from build123d import *

# Parameters (mm, degrees)
SKETCH_1_W             = 56
SKETCH_1_H             = 88
EXTRUDE_1_DEPTH        = 2.7
FILLET_1_R             = 1
SKETCH_8_R             = 1.6
SKETCH_8_R_2           = 1.75
CUT_EXTRUDE_1_DEPTH    = 10
CHAMFER_1_SIZE         = 6
SKETCH_16_R            = 3
EXTRUDE_3_DEPTH        = 1
HOLE_WIZARD_M4_1_D     = 3.3
HOLE_WIZARD_M4_1_DEPTH = 10.1
HOLE_WIZARD_M4_1_TIP   = 0.991420021
SKETCH_11_W            = 6
SKETCH_11_H            = 6
EXTRUDE_2_DEPTH        = 3.3
HOLE_WIZARD_M3_1_D     = 2.5
HOLE_WIZARD_M3_1_DEPTH = 7.5
HOLE_WIZARD_M3_1_TIP   = 0.751075774
SKETCH_14_W            = 30
SKETCH_14_H            = 47
CUT_EXTRUDE_2_DEPTH    = 10
FILLET_2_R             = 2
SKETCH_15_W            = 20
SKETCH_15_H            = 2.7
CUT_EXTRUDE_3_DEPTH    = 5
CHAMFER_2_SIZE         = 0.5
FILLET_3_R             = 2


with BuildPart() as part:
    # 草图1 → 凸台-拉伸1 (new body)
    with BuildSketch(Plane.XY):
        Rectangle(SKETCH_1_W, SKETCH_1_H)
    extrude(amount=EXTRUDE_1_DEPTH)

    # 圆角1
    fillet_1_edges = [part.edges().sort_by_distance(p)[0] for p in [
        (28, -44, 1.35),
        (28, 44, 1.35),
    ]]
    fillet(fillet_1_edges, radius=FILLET_1_R)

    # 草图8 → 切除-拉伸1 (cut)
    with BuildSketch(Plane(origin=(0, 0, 0), x_dir=(-1, 0, 0), z_dir=(0, 0, -1))):
        with Locations((-24, 41)):
            Circle(SKETCH_8_R)
        with Locations((20, 41)):
            Circle(SKETCH_8_R_2)
        with Locations((-24, -41)):
            Circle(SKETCH_8_R)
        with Locations((20, -41)):
            Circle(SKETCH_8_R_2)
    extrude(amount=-CUT_EXTRUDE_1_DEPTH, mode=Mode.SUBTRACT)

    # 倒角1
    chamfer_1_edges = [part.edges().sort_by_distance(p)[0] for p in [
        (-28, -44, 1.35),
        (-28, 44, 1.35),
    ]]
    chamfer(chamfer_1_edges, length=CHAMFER_1_SIZE)

    # 草图16 → 凸台-拉伸3 (add)
    with BuildSketch(Plane(origin=(0, 0, 0), x_dir=(-1, 0, 0), z_dir=(0, 0, -1))):
        with Locations((22.2, -20.7)):
            Circle(SKETCH_16_R)
        with Locations((-20.2, 30.7)):
            Circle(SKETCH_16_R)
    extrude(amount=EXTRUDE_3_DEPTH)

    # M4 螺纹孔1
    with Locations(Plane.XY.offset(2.7)):
        with Locations((20.2, 30.7), (-22.2, -20.7)):
            Hole(HOLE_WIZARD_M4_1_D / 2, depth=HOLE_WIZARD_M4_1_DEPTH)
            with Locations((0, 0, -(HOLE_WIZARD_M4_1_DEPTH + HOLE_WIZARD_M4_1_TIP / 2))):  # 118° drill point
                Cone(0, HOLE_WIZARD_M4_1_D / 2, HOLE_WIZARD_M4_1_TIP, mode=Mode.SUBTRACT)

    # 草图11 → 凸台-拉伸2 (add)
    with BuildSketch(Plane(origin=(0, 0, 0), x_dir=(-1, 0, 0), z_dir=(0, 0, -1))):
        with Locations((-16, 41)):
            Rectangle(SKETCH_11_W, SKETCH_11_H)
        with Locations((12, 41)):
            Rectangle(SKETCH_11_W, SKETCH_11_H)
        with Locations((-16, -41)):
            Rectangle(SKETCH_11_W, SKETCH_11_H)
        with Locations((12, -41)):
            Rectangle(SKETCH_11_W, SKETCH_11_H)
    extrude(amount=EXTRUDE_2_DEPTH)

    # M3 螺纹孔1
    with Locations(Plane(origin=(0, 0, -3.3), x_dir=(-1, 0, 0), z_dir=(0, 0, -1))):
        with Locations((-16, 41), (12, 41), (-16, -41), (12, -41)):
            Hole(HOLE_WIZARD_M3_1_D / 2, depth=HOLE_WIZARD_M3_1_DEPTH)
            with Locations((0, 0, -(HOLE_WIZARD_M3_1_DEPTH + HOLE_WIZARD_M3_1_TIP / 2))):  # 118° drill point
                Cone(0, HOLE_WIZARD_M3_1_D / 2, HOLE_WIZARD_M3_1_TIP, mode=Mode.SUBTRACT)

    # 草图14 → 切除-拉伸2 (cut)
    with BuildSketch(Plane(origin=(0, 0, 0), x_dir=(-1, 0, 0), z_dir=(0, 0, -1))):
        with Locations((7, 7.5)):
            Rectangle(SKETCH_14_W, SKETCH_14_H)
    extrude(amount=-CUT_EXTRUDE_2_DEPTH, mode=Mode.SUBTRACT)

    # 圆角2
    fillet_2_edges = [part.edges().sort_by_distance(p)[0] for p in [
        (8, -16, 1.35),
        (8, 31, 1.35),
        (-22, 31, 1.35),
        (-22, -16, 1.35),
    ]]
    fillet(fillet_2_edges, radius=FILLET_2_R)

    # 草图15 → 切除-拉伸3 (cut)
    with BuildSketch(Plane.XZ.offset(44)):
        with Locations((2, 1.35)):
            Rectangle(SKETCH_15_W, SKETCH_15_H)
    cut_extrude_3 = extrude(amount=-CUT_EXTRUDE_3_DEPTH, mode=Mode.SUBTRACT)

    # 镜向2: 切除-拉伸3 across plane
    add(cut_extrude_3.mirror(Plane(origin=(0, 0, 0), x_dir=(0, 0, 1), z_dir=(0, -1, 0))), mode=Mode.SUBTRACT)

    # 倒角2
    chamfer_2_edges = [part.edges().sort_by_distance(p)[0] for p in [
        (12, -44, 1.35),
        (-8, -44, 1.35),
        (12, 44, 1.35),
        (-8, 44, 1.35),
    ]]
    chamfer(chamfer_2_edges, length=CHAMFER_2_SIZE)

    # 圆角3
    fillet_3_edges = [part.edges().sort_by_distance(p)[0] for p in [
        (19, -38, -1.65),
        (13, -38, -1.65),
        (-9, -38, -1.65),
        (-15, -38, -1.65),
        (19, 38, -1.65),
        (13, 38, -1.65),
        (-9, 38, -1.65),
        (-15, 38, -1.65),
    ]]
    fillet(fillet_3_edges, radius=FILLET_3_R)


solid = part.part
Could you check a few things on this model? Use its own coordinates, in mm. A direction names the side the tool comes from. Round coordinates to 2 decimals unless told otherwise and drop trailing zeros. Write each loop counter-clockwise with the first axis right and the second up, starting at its lowest first coordinate (ties: lowest second). Pieces come first, ordered by that corner, then holes. Notation, with made-up numbers: (-4, -28.75) - (5, -28.75) arc R17 cw to (5, 0.25) - close; hole circle Ø2 at (33, 11.5). An arc over 180 degrees is marked (long way). Put each result on its own line as item: value. Start each with the question number.
(1) I want a section at B-B, the plane x = 16. Please give me the cut outline in (y, z).
(2) Thinking about a two-plate mould opening in X: for faces 1 (the flat face through (-23.5, -22, -1)), 2 (the flat face through (19, 42, -2)), 3 (the cylindrical face through (-13.25, -40.95, -0.26)), 4 (the cylindrical face through (22.41, 32.73, -0.49)), which applies, released by +X, released by -X, zero draft, split by the parting line, or undercut?
(3) I want a section at D-D, the plane x = 4.5. Please give me the cut outline in (y, z), plus the area to 3 significant figures.
(4) I want a section at C-C, the plane y = -41. Give the number of separate pieces and of enclosed holes in the cut face, plus the area to 3 significant figures.
(5) I need wall thicknesses on probe 1 along Y at (x, z) = (-12, -0.95); probe 2 along Y at (x, z) = (24, 1.5); probe 3 along Y at (x, z) = (4.5, 0.2). Which ranges of each line are inside material? Lowest first, please.
(6) I want a section at A-A, the plane y = -20.7. Please give me the cut outline in (x, z), plus the area to 3 significant figures.
(7) Will these pins go through, and if not, where does the flat tip stop? pin 1 (4.5 mm diameter, centred on x = -22.2, y = -20.7, fed in from -Z); pin 2 (2 mm diameter, centred on x = 4.5, z = 0.5, fed in from +Y); pin 3 (1.6 mm diameter, centred on y = -42.5, z = -1.5, fed in from -X).
(8) For faces 5 (the flat face through (-7, -16, 1)), 6 (the cylindrical face through (18.4, 38.57, -1.67)), 7 (the flat face through (-8, -41, 1)), 8 (the flat face through (-15, -42, -2)), which set-ups out of +Z, -Z, +X, -X, +Y, -Y let a thin tool reach every point of the face, with its end or its side?
Here are the results:
1. outline: (-44, -3.3) - (-42.25, -3.3) - (-42.25, 2.7) - (-44, 2.7) - close; (-39.75, -3.3) - (-38, -3.3) - (-38, 0) - (38, 0) - (38, -3.3) - (39.75, -3.3) - (39.75, 2.7) - (-39.75, 2.7) - close; (42.25, -3.3) - (44, -3.3) - (44, 2.7) - (42.25, 2.7) - close
2. face 1: zero draft
2. face 2: released by +X
2. face 3: undercut
2. face 4: split by the parting line
3. outline: (-39, 0) - (-16, 0) - (-16, 2.7) - (-39, 2.7) - close; (31, 0) - (39, 0) - (39, 2.7) - (31, 2.7) - close
3. area: 83.7 mm^2
4. separate pieces: 6
4. enclosed holes: 0
4. area: 80.6 mm^2
5. probe 1: y = -44 to -42.25, -39.75 to -38, 38 to 39.75, 42.25 to 44
5. probe 2: y = -44 to -42.6, -39.4 to 39.4, 42.6 to 44
5. probe 3: y = -39 to -16, 31 to 39
6. outline: (-28, 0) - (-25.2, 0) - (-25.2, -1) - (-23.85, -1) - (-23.85, 2.7) - (-28, 2.7) - close; (-20.55, -1) - (-19.2, -1) - (-19.2, 0) - (28, 0) - (28, 2.7) - (-20.55, 2.7) - close
6. area: 145 mm^2
7. pin 1: stops at z = -1
7. pin 2: stops at y = 39
7. pin 3: stops at x = -15
8. face 5: +Z, -Z
8. face 6: -Z, +X
8. face 7: +Z, -Z, -Y
8. face 8: -Z, -X, +Y, -Y
